For this review, take the finished solid that the model builds, in its own axes (mm). A direction names the side the tool comes from. Give positions to 0.01 mm unless a question says otherwise; leave off trailing zeros. Write each loop counter-clockwise with the first axis right and the second up, starting at its lowest first coordinate (ties: lowest second). Pieces come first, ordered by that corner, then holes.
from build123d import *

# Parameters (mm, degrees)
F1_DEPTH = 20


with BuildPart() as f1:
    # F0 (on Front) → F1 (new body)
    with BuildSketch(Plane.XZ):
        with BuildLine():
            ThreePointArc((-17.147831, -10.293294), (5.34057, -19.273773), (20, 0))
            ThreePointArc((20, 0), (9.493262, 17.603351), (-10.987798, 16.711323))
            ThreePointArc((-10.987798, 16.711323), (-12.232653, 15.54701), (-13.657159, 14.611023))
            ThreePointArc((-13.657159, 14.611023), (-14.240981, 14.042594), (-14.801165, 13.450856))
            ThreePointArc((-14.801165, 13.450856), (-19.593289, 4.012858), (-18.89732, -6.549144))
            ThreePointArc((-18.89732, -6.549144), (-18.803044, -6.815095), (-18.705026, -7.079689))
            ThreePointArc((-18.705026, -7.079689), (-17.574185, -8.515807), (-17.147831, -10.293294))
        make_face()
        Polygon((0, 15), (14.265848, 4.635255), (8.816779, -12.135255), (-8.816779, -12.135255), (-14.265848, 4.635255), align=None, mode=Mode.SUBTRACT)
        with BuildLine():
            ThreePointArc((-13.657159, 14.611023), (-12.232653, 15.54701), (-10.987798, 16.711323))
            ThreePointArc((-10.987798, 16.711323), (-12.367146, 15.717942), (-13.657159, 14.611023))
        make_face()
        with BuildLine():
            ThreePointArc((-18.705026, -7.079689), (-17.998296, -8.721316), (-17.147831, -10.293294))
            ThreePointArc((-17.147831, -10.293294), (-17.574185, -8.515807), (-18.705026, -7.079689))
        make_face()
        with BuildLine():
            ThreePointArc((-14.801165, 13.450856), (-14.240981, 14.042594), (-13.657159, 14.611023))
            ThreePointArc((-13.657159, 14.611023), (-15.505162, 13.839074), (-17.469928, 13.450856))
            Line((-17.469928, 13.450856), (-14.801165, 13.450856))
        make_face()
        with BuildLine():
            ThreePointArc((-19.527159, -6.549144), (-19.100839, -6.79078), (-18.705026, -7.079689))
            ThreePointArc((-18.705026, -7.079689), (-18.803044, -6.815095), (-18.89732, -6.549144))
            Line((-18.89732, -6.549144), (-19.527159, -6.549144))
        make_face()
        with BuildLine():
            ThreePointArc((-18.89732, -6.549144), (-19.593289, 4.012858), (-14.801165, 13.450856))
            Line((-14.801165, 13.450856), (-17.469928, 13.450856))
            ThreePointArc((-17.469928, 13.450856), (-18.416226, 13.405981), (-19.362524, 13.450856))
            Line((-19.362524, 13.450856), (-96.597262, 13.450856))
            ThreePointArc((-96.597262, 13.450856), (-96.773372, 13.449305), (-96.949482, 13.450856))
            Line((-96.949482, 13.450856), (-102.184436, 13.450856))
            ThreePointArc((-102.184436, 13.450856), (-99.806962, 6.911334), (-99, 0))
            ThreePointArc((-99, 0), (-99.181444, -3.294498), (-99.723581, -6.549144))
            Line((-99.723581, -6.549144), (-96.597262, -6.549144))
            Line((-96.597262, -6.549144), (-23.303071, -6.549144))
            ThreePointArc((-23.303071, -6.549144), (-21.415115, -6.108877), (-19.527159, -6.549144))
            Line((-19.527159, -6.549144), (-18.89732, -6.549144))
        make_face()
        with BuildLine():
            Line((-96.333308, 3.450856), (-96.333308, 3.451164))
            ThreePointArc((-96.333308, 3.451164), (-94.849143, 7.006289), (-91.277745, 8.450856))
            Line((-91.277745, 8.450856), (-31.333308, 8.450856))
            ThreePointArc((-31.333308, 8.450856), (-27.797775, 6.98639), (-26.333308, 3.450856))
            ThreePointArc((-26.333308, 3.450856), (-27.797775, -0.084678), (-31.333308, -1.549144))
            Line((-31.333308, -1.549144), (-91.333308, -1.549144))
            ThreePointArc((-91.333308, -1.549144), (-94.868842, -0.084678), (-96.333308, 3.450856))
        make_face(mode=Mode.SUBTRACT)
        with BuildLine():
            ThreePointArc((-19.362524, 13.450856), (-18.416226, 13.405981), (-17.469928, 13.450856))
            Line((-17.469928, 13.450856), (-19.362524, 13.450856))
        make_face()
        with BuildLine():
            Line((-23.303071, -6.549144), (-19.527159, -6.549144))
            ThreePointArc((-19.527159, -6.549144), (-21.415115, -6.108877), (-23.303071, -6.549144))
        make_face()
        with BuildLine():
            ThreePointArc((-96.949482, 13.450856), (-96.773372, 13.449305), (-96.597262, 13.450856))
            Line((-96.597262, 13.450856), (-96.949482, 13.450856))
        make_face()
        with BuildLine():
            ThreePointArc((-99.918438, -7.366324), (-98.293046, -6.814691), (-96.597262, -6.549144))
            Line((-96.597262, -6.549144), (-99.723581, -6.549144))
            ThreePointArc((-99.723581, -6.549144), (-99.818149, -6.958416), (-99.918438, -7.366324))
        make_face()
        with BuildLine():
            Line((-102.184436, 13.450856), (-96.949482, 13.450856))
            ThreePointArc((-96.949482, 13.450856), (-100.721368, 14.261632), (-103.905615, 16.439946))
            ThreePointArc((-103.905615, 16.439946), (-103.002031, 14.970158), (-102.184436, 13.450856))
        make_face()
        with BuildLine():
            ThreePointArc((-99.918438, -7.366324), (-99.818149, -6.958416), (-99.723581, -6.549144))
            ThreePointArc((-99.723581, -6.549144), (-99.181444, -3.294498), (-99, 0))
            ThreePointArc((-99, 0), (-99.806962, 6.911334), (-102.184436, 13.450856))
            ThreePointArc((-102.184436, 13.450856), (-103.002031, 14.970158), (-103.905615, 16.439946))
            ThreePointArc((-103.905615, 16.439946), (-104.859329, 17.565659), (-105.637028, 18.819446))
            ThreePointArc((-105.637028, 18.819446), (-159, 0), (-105.637028, -18.819446))
            ThreePointArc((-105.637028, -18.819446), (-104.850555, -12.057916), (-99.918438, -7.366324))
        make_face()
        Polygon((-117.452995, 20), (-105.905989, 0), (-117.452995, -20), (-140.547005, -20), (-152.094011, 0), (-140.547005, 20), align=None, mode=Mode.SUBTRACT)
        with BuildLine():
            ThreePointArc((-105.637028, -18.819446), (-102.159717, -13.401463), (-99.918438, -7.366324))
            ThreePointArc((-99.918438, -7.366324), (-104.850555, -12.057916), (-105.637028, -18.819446))
        make_face()
        with BuildLine():
            ThreePointArc((-105.637028, 18.819446), (-104.859329, 17.565659), (-103.905615, 16.439946))
            ThreePointArc((-103.905615, 16.439946), (-104.742128, 17.650939), (-105.637028, 18.819446))
        make_face()
    extrude(amount=F1_DEPTH)


solid = f1.part
(1) Tool access review of faces 1 (the flat face through (-59, -10, -6.549)), 2 (the flat face through (-111.76, -9.86, 10.14)), 3 (the flat face through (-57, -10, 13.451)): name each direction out of +Z, -Z, +X, -X, +Y, -Y from which nothing blocks a thin tool from reaching the whole face with its end or side.
(2) For L1, parallel to X at y = -15.25, z = -3 (3 decimals); L2, parallel to X at y = -4, z = -2.5; L3, parallel to X at y = -13.75, z = -10.5, list the stretches that pass through material, from the lowest coordinate up.
(3) We need section C-C (x = -36.5). Write out the cut boundary in (y, z).
(4) We need section A-A (x = -129). Write out the cut boundary in (y, z).
(5) Clearance check with flat-ended pins moving along their axes: pin 1 Ø2 at (x, y) = (-98.5, -9.5) entering from +Z; pin 2 Ø6 at (x, y) = (-53, -8) entering from +Z; pin 3 Ø5 at (y, z) = (-17, 8.5) entering from +X. State where each tip first meets the part, or that it passes through.
(6) The part is to be moulded in two halves that separate along Z. For faces 4 (the flat face through (-83, 0, -4)), 5 (the flat face through (-111.6, -9.86, -9.86)), 6 (the cylindrical face through (-18.01, -9.86, -8.7)), 7 (the cylindrical face through (-100.67, -9.86, 14.24)), say which applies: +Z half, -Z half, draft (parallel to the pull), parting line (faces both ways), or undercut.
(7) We need section B-B (y = -8.75). Count the separate pieces of the cut face and the enclosed holes in it, and give its area (3 significant figures).
The answers:
1. face 1: -Z, +Y, -Y
1. face 2: +Y, -Y
1. face 3: +Z, +Y, -Y
2. L1: x = -158.85 to -150.362, -107.638 to -11.785, 11.785 to 19.774
2. L2: x = -158.9 to -150.65, -107.35 to -11.95, 11.95 to 19.84
2. L3: x = -157.1 to -146.03, -111.97 to -100.9, -17.02 to -9.35, 9.35 to 17.02
3. outline: (-20, -6.55) - (0, -6.55) - (0, -1.55) - (-20, -1.55) - close; (-20, 8.45) - (0, 8.45) - (0, 13.45) - (-20, 13.45) - close
4. outline: (-20, -30) - (0, -30) - (0, -20) - (-20, -20) - close; (-20, 20) - (0, 20) - (0, 30) - (-20, 30) - close
5. pin 1: stops at z = 13.83
5. pin 2: stops at z = 13.45
5. pin 3: stops at x = 19.08
6. face 4: draft
6. face 5: undercut
6. face 6: -Z half
6. face 7: +Z half
7. separate pieces: 1
7. enclosed holes: 3
7. area: 3,110 mm2
